For this review, take the finished solid that the model builds, in its own axes (mm). A direction names the side the tool comes from. Coordinates: 2 decimals unless noted, no trailing zeros. Order: outer loops, then holes, each group sorted by start corner. A loop starts at its lowest first (then second) coordinate and runs counter-clockwise, first axis right, second up. Notation, with made-up numbers: (-37, -2.75) - (20, -2.75) arc R27 ccw to (20, 34.25) - close; hole circle Ø7 at (-2.5, -3). An arc over 180 degrees is marked (long way). One line per item, written item: value. Start each with the question number.
(1) Mouldability with a two-part tool opening along Z and no side actions: class faces 4 (the flat face through (1, 0, -20)), 5 (the flat face through (10, 165, 0)), 6 (the flat face through (18.5, 175, -20)) as released by +Z, released by -Z, zero draft, split by the parting line, or undercut.
(2) Consider section B-B on x = 7.25. Write out the cut boundary in (y, z).
(3) To check wall thickness, follow line 1 along X through (y, z) = (147, -3); line 2 along Z through (x, y) = (16.25, 37); line 3 along Y through (x, z) = (19.25, -28.5). State the ranges of each line that lie inside material, in increasing order.
(4) Consider section C-C on y = 166.5. Write out the cut boundary in (x, z).
(5) Consider section A-A on z = -34. Write out the cut boundary in (x, y).
(6) For faces 1 (the flat face through (19, 20, -21)), 2 (the flat face through (11, 334, -1)), 3 (the flat face through (10, 165, -38.5)), list the 3-axis set-ups (+Z, -Z, +X, -X, +Y, -Y) from which the entire face can be reached by the end or side of a thin tool; tool diameter is ignored.
(7) Clearance check with flat-ended pins moving along their axes: pin 1 (1.6 mm diameter, centred on y = 12, z = -39.5, fed in from +X); pin 2 (0.8 mm diameter, centred on x = 19.5, z = -17.5, fed in from +Y). State where each tip first meets the part, or that it passes through.
```python
from build123d import *

# Parameters (mm, degrees)
SKETCH1_W           = 17
SKETCH1_H           = 37
BOSS_EXTRUDE1_DEPTH = 334
SKETCH2_W           = 10
SKETCH2_H           = 20
CUT_EXTRUDE1_DEPTH  = 40
SKETCH4_W           = 10
SKETCH4_H           = 8
CUT_EXTRUDE3_DEPTH  = 337.980711614


with BuildPart() as part:
    # Sketch1 → Boss-Extrude1 (new body)
    with BuildSketch(Plane(origin=(0, 0, 0), x_dir=(1, 0, 0), z_dir=(0, 1, 0))):
        with BuildLine():
            Line((0.5, 0), (19.5, 0))
            ThreePointArc((19.5, 0), (19.853553391, 0.146446609), (20, 0.5))
            Line((20, 0.5), (20, 39.5))
            ThreePointArc((20, 39.5), (19.853553391, 39.853553391), (19.5, 40))
            Line((19.5, 40), (0.5, 40))
            ThreePointArc((0.5, 40), (0.146446609, 39.853553391), (0, 39.5))
            Line((0, 39.5), (0, 0.5))
            ThreePointArc((0, 0.5), (0.146446609, 0.146446609), (0.5, 0))
        make_face()
        with Locations((10, 20)):
            Rectangle(SKETCH1_W, SKETCH1_H, mode=Mode.SUBTRACT)
    extrude(amount=BOSS_EXTRUDE1_DEPTH)

    # Sketch2 → Cut-Extrude1 (cut)
    with BuildSketch(Plane.XY):
        with Locations((15, 10)):
            Rectangle(SKETCH2_W, SKETCH2_H)
    extrude(amount=-CUT_EXTRUDE1_DEPTH, mode=Mode.SUBTRACT)

    # Sketch4 → Cut-Extrude3 (cut, through all)
    with BuildSketch(Plane(origin=(20, 0, 0), x_dir=(0, 0, -1), z_dir=(1, 0, 0))):
        with Locations((16.16, 330)):
            Rectangle(SKETCH4_W, SKETCH4_H)
    extrude(amount=-CUT_EXTRUDE3_DEPTH, mode=Mode.SUBTRACT)


solid = part.part
```
Geometry check:
1. face 4: zero draft
1. face 5: released by +Z
1. face 6: undercut
2. outline: (0, -40) - (334, -40) - (334, -38.5) - (0, -38.5) - close; (0, -1.5) - (334, -1.5) - (334, 0) - (0, 0) - close
3. line 1: x = 0 to 1.5, 18.5 to 20
3. line 2: z = -40 to -38.5, -1.5 to 0
3. line 3: y = 20 to 334
4. outline: (0, -39.5) arc R0.5 ccw to (0.5, -40) - (19.5, -40) arc R0.5 ccw to (20, -39.5) - (20, -0.5) arc R0.5 ccw to (19.5, 0) - (0.5, 0) arc R0.5 ccw to (0, -0.5) - close; hole (1.5, -38.5) - (18.5, -38.5) - (18.5, -1.5) - (1.5, -1.5) - close
5. outline: (0, 0) - (1.5, 0) - (1.5, 334) - (0, 334) - close; (18.5, 20) - (20, 20) - (20, 334) - (18.5, 334) - close
6. face 1: +Z, -Z, +X, -Y
6. face 2: +Z, -Z, +X, -X, +Y
6. face 3: +Y, -Y
7. pin 1: stops at x = 10
7. pin 2: stops at y = 326
